Work out the finished part from the listing and answer in its coordinate system (mm). A direction names the side the tool comes from. Coordinates: 2 decimals unless noted, no trailing zeros. Order: outer loops, then holes, each group sorted by start corner. A loop starts at its lowest first (then second) coordinate and runs counter-clockwise, first axis right, second up. Notation, with made-up numbers: (71, 29) - (125, 29) arc R29 ccw to (125, 51) - close; hole circle Ø9 at (2.5, -18). An arc over 180 degrees is marked (long way). Answer as a JSON object with one key per item and string values. Group by question number.
1) Section A-A (z = 3) is taken. Give the vertices of the cut face in (x, y), plus the area to 3 significant figures.
2) This flat-tipped pin is pushed along its axis until it touches: P1, Ø3, axis at y = -2, z = 17, coming from the +X side. Where does it stop, or does it pass through?
3) Find the intervals of material crossed by line 1 along Y through (x, z) = (0, 6.5); line 2 along Y through (x, z) = (0.5, 19); line 3 along Z through (x, y) = (1.75, -1.75), in increasing order.
4) Section B-B (z = -1.5) is taken. Give the vertices of the cut face in (x, y).
5) The mould has two halves that part along X. Classify faces 1 (the face through (-1, 1, 25.7)), 2 (the face through (0, 0, 0)): released by +X, released by -X, zero draft, split by the parting line, or undercut.
6) A tool of negligible diameter and unlimited length cuts with its end or side. For faces 3 (the face through (-1.19, -0.38, 12.67)), 4 (the face through (-1.72, -2.7, 12.67)), from which of +Z, -Z, +X, -X, +Y, -Y can it reach the whole face along a straight path? Write none if from no direction.
from build123d import *

# Parameters (mm, degrees)
SKETCH3_R                 = 3.2
BOSS_EXTRUDE2_DEPTH       = 25.7
CUT_EXTRUDE1_DEPTH        = 27.095401894
CUT_EXTRUDE1_DEPTH_BACK   = 25.7
SKETCH6_R                 = 1.25
TAP_DRILL_FOR_4_40_TAP1_D = 2.2606


with BuildPart() as part:
    # Sketch3 → Boss-Extrude2 (new body)
    with BuildSketch(Plane.XY):
        with Locations(Location((0, 0, 0), (0, 0, 180))):
            Circle(SKETCH3_R)
    extrude(amount=BOSS_EXTRUDE2_DEPTH)

    # Sketch6 → Cut-Extrude1 (cut, two sides: drawn at the far end of the back side and taken through both)
    with BuildSketch(Plane.XY.offset(25.7).offset(-CUT_EXTRUDE1_DEPTH_BACK)):
        with Locations(Location((0, 0, 0), (0, 0, 180))):
            Circle(SKETCH6_R)
    extrude(amount=CUT_EXTRUDE1_DEPTH + CUT_EXTRUDE1_DEPTH_BACK, mode=Mode.SUBTRACT)

    # Sketch7 → Revolve1 (revolve)
    with BuildSketch(Plane(origin=(0, 0, 0), x_dir=(1, 0, 0), z_dir=(0, 1, 0)), mode=Mode.PRIVATE) as revolve1_sk:
        Polygon((0, 0), (-3.2, 0), (0, 5.5), align=None)
    revolve(revolve1_sk.sketch.rotate(Axis((0, 0, -5.5), (0, 0, 1)), 180), axis=Axis((0, 0, -5.5), (0, 0, 1)))

    # Tap Drill for #4-40 Tap1 (through all)
    with Locations(Plane(origin=(3.187528357, -0.282246299, 21.7), x_dir=(0.088201968553, 0.996102611553, 0), z_dir=(0.996102611553, -0.088201968553, 0))):
        with Locations((0, 0)):
            Hole(TAP_DRILL_FOR_4_40_TAP1_D / 2)


solid = part.part
Report:
{
 "1": {"outline": "circle Ø6.4 at (0, 0); hole circle Ø2.5 at (0, 0)", "area": "27.3 mm²"},
 "2": {"P1": "stops at x = 3.16"},
 "3": {"line 1": "y = -3.2 to -1.25, 1.25 to 3.2", "line 2": "y = -3.16 to -1.15, 1.15 to 3.16", "line 3": "z = -1.25 to 25.7"},
 "4": {"outline": "circle Ø4.65 at (0, 0)"},
 "5": {"face 1": "zero draft", "face 2": "undercut"},
 "6": {"face 3": "+Z", "face 4": "+Z, -Z"}
}
